from build123d import *

# Parameters (mm, degrees)
SKETCH3_R           = 25
BOSS_EXTRUDE1_DEPTH = 310
SKETCH6_R           = 20
CUT_EXTRUDE2_DEPTH  = 330


with BuildPart() as part:
    # Sketch1 → Revolve1 (revolve)
    with BuildSketch(Plane.XY, mode=Mode.PRIVATE) as revolve1_sk:
        with BuildLine():
            Line((5, 0), (0, 0))
            ThreePointArc((0, 0), (87.867965644, 212.132034356), (300, 300))
            Line((300, 300), (300, 295))
            ThreePointArc((300, 295), (91.40349955, 208.59650045), (5, 0))
        make_face()
    revolve(revolve1_sk.sketch.rotate(Axis((300, 300, 0), (0, -1, 0)), 180), axis=Axis((300, 300, 0), (0, -1, 0)))

    # Sketch3 → Boss-Extrude1 (add)
    with BuildSketch(Plane(origin=(0, 0, 0), x_dir=(1, 0, 0), z_dir=(0, 1, 0))):
        with Locations(Location((300, 0, 0), (0, 0, 270))):
            Circle(SKETCH3_R)
    extrude(amount=BOSS_EXTRUDE1_DEPTH)

    # Sketch5 → Cut-Revolve1 (revolve, cut)
    with BuildSketch(Plane.XY, mode=Mode.PRIVATE) as cut_revolve1_sk:
        with BuildLine():
            Line((300.755316248, 295.755316248), (300.755316248, 0))
            Line((300.755316248, 0), (5, 0))
            ThreePointArc((5, 0), (91.624726557, 209.130589691), (300.755316248, 295.755316248))
        make_face()
    revolve(cut_revolve1_sk.sketch.rotate(Axis((300.755316248, 295.755316248, 0), (0, -1, 0)), 180), axis=Axis((300.755316248, 295.755316248, 0), (0, -1, 0)), mode=Mode.SUBTRACT)

    # Sketch6 → Cut-Extrude2 (cut)
    with BuildSketch(Plane(origin=(0, 310, 0), x_dir=(1, 0, 0), z_dir=(0, 1, 0))):
        with Locations(Location((300, 0, 0), (0, 0, 270))):
            Circle(SKETCH6_R)
    extrude(amount=-CUT_EXTRUDE2_DEPTH, mode=Mode.SUBTRACT)


solid = part.part
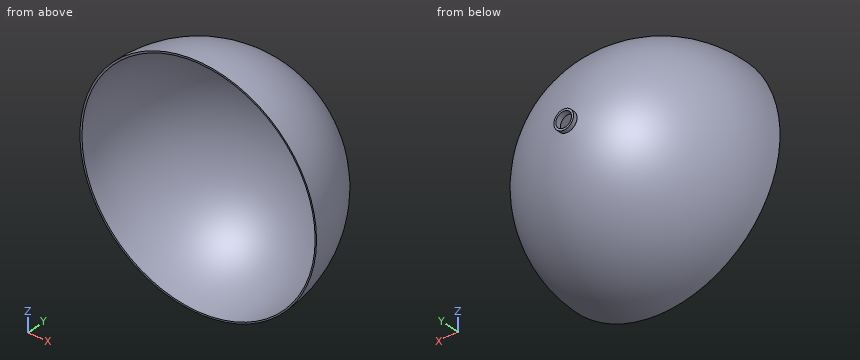
Part model, mm, in its own coordinate system. Coordinates: 2 decimals unless noted, no trailing zeros. Loops run counter-clockwise (first coordinate to the right, second up) from the corner with the lowest first, then second, coordinate; pieces in that order, holes last. Notation, with made-up numbers: (36, -34.5) -> (79, -34.5) arc R24 cw to (79, -15.5) -> close; hole circle Ø7 at (42.5, 71.25). An arc over 180 degrees is marked (long way). Use a Markdown table: item, result. Add a question column.
Item 1: Band-saw the part on C-C on y = 84. Write the cut outline in (x, z).
Item 2: Band-saw the part on A-A on z = 0. Write the cut outline in (x, y).
Item 3: Probe probe 1 along X at (y, z) = (300, 0); probe 2 along Z at (x, y) = (300, 303.5); probe 3 along X at (y, z) = (187, -135). List the from-to ranges inside material, lowest first.
Item 4: Flat gauge pins, fed straight in: P1, Ø1.5, axis at y = 129.5, z = -110, coming from the +X side; P2, Ø1, axis at y = 65, z = 213.5, coming from the +X side; P3, Ø4, axis at x = 165, z = -228, coming from the +Y side. Where does each tip first touch, or does it go through?
Item 5: Band-saw the part on B-B on x = 300. Write the cut outline in (y, z).
Item 6: Band-saw the part on D-D on z = -163. Write the cut outline in (x, y), plus the area to 3 significant figures.
Geometry says:
| question | item | result |
|---|---|---|
| 1 | outline | circle Ø576 at (300, 0); hole circle Ø567.15 at (300.76, 0) |
| 2 | outline | (0, 0) -> (5, 0) arc R295.76 cw to (280, 295.03) -> (280, 310) -> (275, 310) -> (275, 298.96) arc R300 ccw to start; (320, 295.13) arc R295.76 cw to (596.51, 0) -> (600, 0) arc R300 ccw to (325, 298.96) -> (325, 310) -> (320, 310) -> close |
| 3 | probe 1 | 275 to 280, 320 to 325 |
| 3 | probe 2 | -25 to -20, 20 to 25 |
| 3 | probe 3 | 108.15 to 115.61, 485.9 to 491.85 |
| 4 | P1 | x = 547.76 |
| 4 | P2 | x = 501.04 |
| 4 | P3 | y = 144.38 |
| 5 | outline | (0, -300) arc R300 ccw to (298.96, -25) -> (310, -25) -> (310, -20) -> (295.08, -20) arc R295.75 cw to (0, -295.75) -> close; (0, 295.75) arc R295.75 cw to (295.08, 20) -> (310, 20) -> (310, 25) -> (298.96, 25) arc R300 ccw to (0, 300) -> close |
| 6 | outline | (48.14, 0) -> (53.97, 0) arc R246.78 cw to (547.54, 0) -> (551.86, 0) arc R251.86 ccw to start |
| 6 | area | 3,970 mm² |
